The model under review builds one solid part; all positions refer to its coordinate system, in mm. Face numbers are marked on the shaded views. A direction names the side the tool comes from. Round coordinates to 2 decimals unless told otherwise and drop trailing zeros. Loops run counter-clockwise (first coordinate to the right, second up) from the corner with the lowest first, then second, coordinate; pieces in that order, holes last. Notation, with made-up numbers: (-10.75, -39.75) - (16.25, -39.75) arc R22 ccw to (16.25, -2.75) - close; hole circle Ø5 at (76.25, 88). An arc over 180 degrees is marked (long way). Answer as CSV lines item,"result".
Autodesk Inventor part; units mm, degrees
ref_plane "YZ Plane" through (0, 0, 0) normal (1, 0, 0) x (0, 1, 0)
ref_plane "XZ Plane" through (0, 0, 0) normal (0, 1, 0) x (-1, 0, 0)
ref_plane "XY Plane" through (0, 0, 0) normal (0, 0, 1) x (1, 0, 0)
sketch "Sketch1" plane through (0, 0, 0) normal (0, 0, 1) x (1, 0, 0)
  circle A0 centre (0, 0) radius 90
  circle A1 centre (0, 0) radius 35
  line L0 (-75, 90) -> (75, 90)
  line L1 (90, 75) -> (90, -75)
  line L2 (75, -90) -> (-75, -90)
  line L3 (-90, -75) -> (-90, 75)
  line L4 (-90, 90) -> (90, -90) construction
  line L5 (90, 90) -> (-90, -90) construction
  arc A2 (-75, 90) -> (-90, 75) centre (-75, 75) ccw
  arc A3 (90, 75) -> (75, 90) centre (75, 75) ccw
  arc A4 (75, -90) -> (90, -75) centre (75, -75) ccw
  arc A5 (-90, -75) -> (-75, -90) centre (-75, -75) ccw
  circle A6 centre (75, 75) radius 4.25
  circle A7 centre (75, -75) radius 4.25
  circle A8 centre (-75, -75) radius 4.25
  circle A9 centre (-75, 75) radius 4.25
  point P0 (0, 90)
  point P1 (90, 0)
  point P2 (0, -90)
  point P3 (-90, 0)
  dimension "d0" = 180
  dimension "d1" = 70
  dimension "d2" = 15
  dimension "d3" = 8.5
extrude "Extrusion1" add sketch "Sketch1" along normal blind 10 contours A0 | A1
extrude "Extrusion2" add sketch "Sketch1" along normal blind 5 contours L1 A4 L2 A0 | A0 L0 A3 L1 | A0 L3 A2 L0 | L2 A5 L3 A0
sketch "Sketch2" plane through (0, 0, 10) normal (0, 0, 1) x (1, 0, 0)
  circle A0 centre (0, 0) radius 35
  dimension "d8" = 70
extrude "Extrusion3" cut sketch "Sketch2" against normal blind 6.5
sketch "Sketch3" plane through (0, 0, 0) normal (0, 0, -1) x (-1, 0, 0)
  circle A0 centre (-75, 75) radius 4.25
  circle A1 centre (75, 75) radius 4.25
  circle A2 centre (-75, -75) radius 4.25
  circle A3 centre (75, -75) radius 4.25
  line L0 (-90, -75) -> (-90, 75)
  arc A4 (-90, -75) -> (-75, -90) centre (-75, -75) ccw
  line L1 (75, -90) -> (-75, -90)
  arc A5 (75, -90) -> (90, -75) centre (75, -75) ccw
  line L2 (90, 75) -> (90, -75)
  arc A6 (90, 75) -> (75, 90) centre (75, 75) ccw
  line L3 (-75, 90) -> (75, 90)
  arc A7 (-75, 90) -> (-90, 75) centre (-75, 75) ccw
  point P0 (0, 0)
extrude "Extrusion4" add sketch "Sketch3" along normal blind 5
sketch "Sketch4" plane through (0, 0, 3.5) normal (0, 0, 1) x (1, 0, 0)
  circle A0 centre (0, 0) radius 35
  circle A1 centre (0, 0) radius 25
  dimension "d13" = 50
extrude "Extrusion5" cut sketch "Sketch4" against normal blind 5 contours A1
sketch "Sketch5" plane through (0, 0, -5) normal (0, 0, -1) x (-1, 0, 0)
  circle A0 centre (10.3923, 6) radius 1.621
  circle A1 centre (0, -12) radius 1.621
  circle A2 centre (-10.3923, 6) radius 1.621
  circle A3 centre (0, 0) radius 4
  circle A4 centre (0, 0) radius 15
  circle A5 centre (10.3923, 6) radius 2
  circle A6 centre (-10.3923, 6) radius 2
  circle A7 centre (0, -12) radius 2
  dimension "d23" = 4
  dimension "d24" = 4
  dimension "d25" = 4
hole "Hole1" at (10.3923, 6, -5) at (-10.3923, 6, -5) at (0, -12, -5) direction (0, 0, 1) diameter 4.2 end through all countersink diameter 9.4 countersink angle 90
properties part number "base onderkant" material "Aluminum 6061"
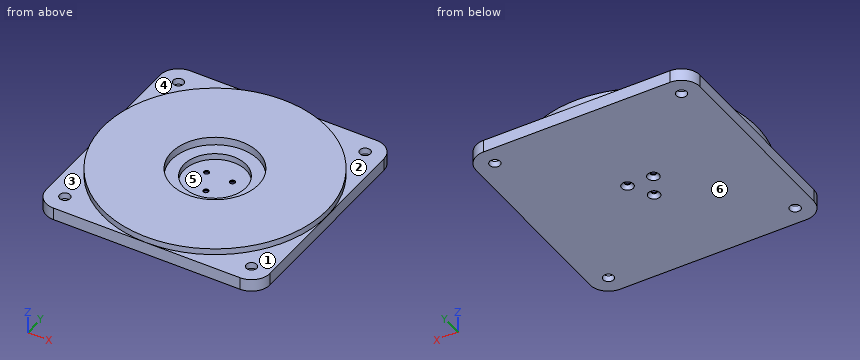
1. Clearance check with flat-ended pins moving along their axes: pin 1 (1.5 mm diameter, centred on x = -14.5, z = 5.5, fed in from +Y); pin 2 (10 mm diameter, centred on x = 75, y = 75, fed in from +Z); pin 3 (1 mm diameter, centred on y = -17, z = 7, fed in from -X); pin 4 (25 mm diameter, centred on x = -1.5, y = -10.5, fed in from +Z). State where each tip first meets the part, or that it passes through.
Numbers:
pin 1,"stops at y = 90"
pin 2,"stops at z = 5"
pin 3,"stops at x = -88.47"
pin 4,"stops at z = -1.5"
2. Wall thickness on probe 1 along X at (y, z) = (6, -2); probe 2 along X at (y, z) = (75, 2.4): over which ranges is each line inside the solid? List them lowest first.
Numbers:
probe 1,"x = -90 to -12.49, -8.29 to 8.29, 12.49 to 90"
probe 2,"x = -90 to -79.25, -70.75 to 70.75, 79.25 to 90"
3. Draft analysis for pull direction Y (two halves, no side actions). For the marked faces 5 and 6, state which applies: +Y half, -Y half, draft (parallel to the pull), parting line (faces both ways), or undercut.
Numbers:
face 5,"undercut"
face 6,"draft"
4. Take a section at C-C (y = -37.5). State the section outline as (x, z) points, plus the area to 3 significant figures.
Numbers:
outline,"(-90, -5) - (90, -5) - (90, 5) - (81.82, 5) - (81.82, 10) - (-81.82, 10) - (-81.82, 5) - (-90, 5) - close"
area,"2,620 mm²"
5. Tool access review of the marked faces 1, 2, 3 and 4: name each direction out of +Z, -Z, +X, -X, +Y, -Y from which nothing blocks a thin tool from reaching the whole face with its end or side.
Numbers:
face 1,"+Z, +X, -Y"
face 2,"+Z, +X, +Y"
face 3,"+Z, -X, -Y"
face 4,"+Z, -X, +Y"
6. Take a section at B-B (x = 68). State the section outline as (y, z) points.
Numbers:
outline,"(-90, -5) - (90, -5) - (90, 5) - (58.96, 5) - (58.96, 10) - (-58.96, 10) - (-58.96, 5) - (-90, 5) - close"
7. Take a section at A-A (y = 6). State the section outline as (x, z) points, plus the area to 3 significant figures.
Numbers:
outline,"(-90, -5) - (-15.09, -5) - (-12.49, -2.4) - (-12.49, -1.5) - (-24.27, -1.5) - (-24.27, 3.5) - (-34.48, 3.5) - (-34.48, 10) - (-89.8, 10) - (-89.8, 5) - (-90, 5) - close; (-8.29, -2.4) - (-5.69, -5) - (5.69, -5) - (8.29, -2.4) - (8.29, -1.5) - (-8.29, -1.5) - close; (12.49, -2.4) - (15.09, -5) - (90, -5) - (90, 5) - (89.8, 5) - (89.8, 10) - (34.48, 10) - (34.48, 3.5) - (24.27, 3.5) - (24.27, -1.5) - (12.49, -1.5) - close"
area,"1,960 mm²"
